from build123d import *

# Parameters (mm, degrees)
F2_R     = 8.189749857
F3_DEPTH = 25
F5_DEPTH = 12.5


with BuildPart() as f1:
    # F0 (on Front) → F1 (revolve)
    with BuildSketch(Plane.XZ):
        Polygon((0, 12.1819740161), (-50, 12.1819740161), (-50, 0), (50, 0), (50, 12.1819740161), align=None)
    revolve(axis=Axis((74.9588809907, 0, 0), (-1, 0, 0)))

    # F2 (on Front) → F3 (join, symmetric)
    with BuildSketch(Plane.XZ):
        with BuildLine():
            Line((-50, -30), (-50, 30))
            add(Edge.make_bspline(
                [(-50, 30), (-73.5387891531, 20), (-105.7427436113, 0), (-73.5387891531, -20), (-50, -30)],
                knots=[0, 0, 0, 0, 0.5, 1, 1, 1, 1], degree=3))
        make_face()
        with Locations((-68.91708076, 0)):
            Circle(F2_R, mode=Mode.SUBTRACT)
        with BuildLine():
            add(Edge.make_bspline(
                [(50, 30), (73.5387891531, 20), (105.7427436113, 0), (73.5387891531, -20), (50, -30)],
                knots=[0, 0, 0, 0, 0.5, 1, 1, 1, 1], degree=3))
            Line((50, 30), (50, -30))
        make_face()
        with Locations((68.91708076, 0)):
            Circle(F2_R, mode=Mode.SUBTRACT)
    extrude(amount=F3_DEPTH, both=True)

    # F4 (on Front) → F5 (cut, symmetric)
    with BuildSketch(Plane.XZ):
        with BuildLine():
            Line((-55, -27.8246053089), (-55, 27.8246053089))
            add(Edge.make_bspline(
                [(-55, 27.8246053089), (-75.7893328005, 18.5497368726), (-103.492199964, -1e-10), (-75.7893328003, -18.5497368728), (-54.9999999995, -27.8246053091)],
                knots=[0.0362565782, 0.0362565782, 0.0362565782, 0.0362565782, 0.5, 0.9637434218, 0.9637434218, 0.9637434218, 0.9637434218], degree=3))
        make_face()
        with BuildLine():
            add(Edge.make_bspline(
                [(55, 27.8246053089), (75.7893328005, 18.5497368726), (103.492199964, -1e-10), (75.7893328003, -18.5497368728), (54.9999999995, -27.8246053091)],
                knots=[0.0362565782, 0.0362565782, 0.0362565782, 0.0362565782, 0.5, 0.9637434218, 0.9637434218, 0.9637434218, 0.9637434218], degree=3))
            Line((55, 27.8246053089), (55, -27.8246053089))
        make_face()
    extrude(amount=F5_DEPTH, both=True, mode=Mode.SUBTRACT)


solid = f1.part
Geometry: final body of the model. Coordinates: model frame, mm. A direction names the side the tool comes from. Round coordinates to 2 decimals unless told otherwise and drop trailing zeros. Write each loop counter-clockwise with the first axis right and the second up, starting at its lowest first coordinate (ties: lowest second). Pieces come first, ordered by that corner, then holes. Notation, with made-up numbers: M -8,54 L 38,54 A5 cw 38,58 Z; hole C 80,47 d1. An arc over 180 degrees is marked long. Write item = value, one per line.
Item 1: Material intervals for line 1 along X through (y, z) = (-15.75, 0); line 2 along X through (y, z) = (10.5, 10.5); line 3 along Y through (x, z) = (75, -6.5), sorted ascending. Write a range as [from, to].
Findings:
line_1 = [-89.64, -77.11], [-60.73, -50], [50, 60.73], [77.11, 89.64]
line_2 = [-55, -50], [50, 55]
line_3 = [-25, -12.5], [12.5, 25]
Item 2: Pin query (flat end, axial travel): P1, Ø1.5, axis at y = -7.5, z = -6.5, coming from the +X side; P2, Ø14.5, axis at x = -68.92, z = 0, coming from the +Y side; P3, Ø5, axis at y = 18, z = 22.5, coming from the -X side; P4, Ø10, axis at x = 25, z = -13.5, coming from the -Y side. Return the tip coordinate at first contact, or that it passes through.
Findings:
P1 = 55
P2 = through
P3 = -70.74
P4 = -8.73
Item 3: Section query B-B on x = 9. Return loops of the section in (y, z).
Findings:
outline = C 0,0 d24.36
Item 4: Access query for faces 4 (the face through (-63, -12.5, -6)), 5 (the face through (63, 12.5, -6)), 6 (the face through (60, -25, 0)). Directions: +Z, -Z, +X, -X, +Y, -Y. A direction counts if a zero-diameter tool reaches every point of the face in a straight line with its end or side. Return the directions, or none.
Findings:
face_4 = +Z, -Z, -X
face_5 = +Z, -Z, +X
face_6 = +Z, -Z, +X, -X, -Y
Item 5: Pull-direction query (Z, two-part tool) for faces 1 (the face through (60, 25, 0)), 2 (the face through (-77.1, -18.66, 0.36)), 3 (the face through (-0.7, 0.54, -12.17)); classes: pulls with the +Z half, pulls with the -Z half, needs draft (parallel to the pull), parting line crosses it, or undercut.
Findings:
face_1 = needs draft
face_2 = undercut
face_3 = parting line crosses it
Item 6: Section query A-A on z = 0. State how many separate pieces and enclosed holes the cut face has, then the cut area to 3 significant figures.
Findings:
separate_pieces = 5
enclosed_holes = 0
area = 3,850 mm^2
